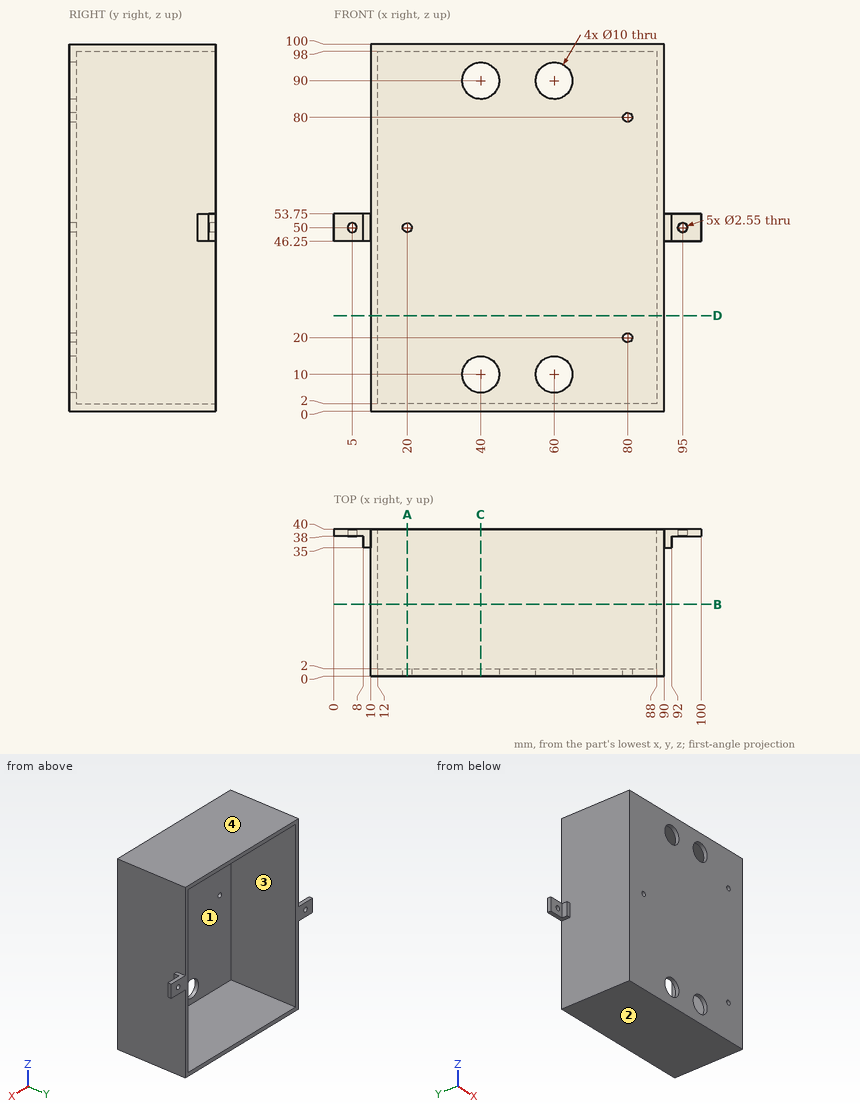
Print and shaded views of the part. All mm, measured from the part's lowest x, y and z. A direction names the side the tool comes from. Coordinates: 2 decimals unless noted, no trailing zeros. Order: outer loops, then holes, each group sorted by start corner. A loop starts at its lowest first (then second) coordinate and runs counter-clockwise, first axis right, second up.
Item 1: Drill centre lines: L1, parallel to Z at x = 40, y = 1; L2, parallel to Z at x = 5, y = 39.35 (3 decimals); L3, parallel to Z at x = 71, y = 34. Where is each one in solid material? Low to high.
Filled in:
L1: z = 0 to 5, 15 to 85, 95 to 100
L2: z = 46.25 to 48.725, 51.275 to 53.75
L3: z = 0 to 2, 98 to 100
Item 2: Saw through at B-B on y = 19.5. List the corners of the cut face in (x, z).
Filled in:
outline: (10, 0) - (90, 0) - (90, 100) - (10, 100) - close; hole (12, 2) - (88, 2) - (88, 98) - (12, 98) - close
Item 3: Tool access for the marked faces 1 and 2: list every direction of +Z, -Z, +X, -X, +Y, -Y with a clear straight run to the whole face (end or side of a thin tool).
Filled in:
face 1: +Y
face 2: -Z, +X, -X, +Y, -Y
Item 4: Saw through at C-C on x = 40. List the corners of the cut face in (y, z).
Filled in:
outline: (0, 0) - (40, 0) - (40, 2) - (2, 2) - (2, 5) - (0, 5) - close; (0, 15) - (2, 15) - (2, 85) - (0, 85) - close; (0, 95) - (2, 95) - (2, 98) - (40, 98) - (40, 100) - (0, 100) - close
Item 5: Saw through at A-A on x = 20. List the corners of the cut face in (y, z) (3 decimals).
Filled in:
outline: (0, 0) - (40, 0) - (40, 2) - (2, 2) - (2, 48.725) - (0, 48.725) - close; (0, 51.275) - (2, 51.275) - (2, 98) - (40, 98) - (40, 100) - (0, 100) - close
Item 6: Saw through at D-D on z = 26. List the corners of the cut face in (x, y).
Filled in:
outline: (10, 0) - (90, 0) - (90, 40) - (88, 40) - (88, 2) - (12, 2) - (12, 40) - (10, 40) - close
Item 7: Mould opens along X. For the marked faces 3 and 4 say: released by +X, released by -X, zero draft, split by the parting line, or undercut.
Filled in:
face 3: undercut
face 4: zero draft
Item 8: Drop flat-ended pins along their axis: pin 1 Ø2 at (x, y) = (15, 25) entering from -Z; pin 2 Ø3 at (x, z) = (95, 50) entering from -Y; pin 3 Ø12 at (y, z) = (6.5, 56) entering from -X; pin 4 Ø1.5 at (y, z) = (37, 48) entering from -X. Give the stop position or say it passes through.
Filled in:
pin 1: stops at z = 0
pin 2: stops at y = 38
pin 3: stops at x = 10
pin 4: stops at x = 8
